Check sheet for the drawn part. Datum: minimum x, y, z corner. Units: mm. Coordinates: 2 decimals unless noted, no trailing zeros. Order: outer loops, then holes, each group sorted by start corner. A loop starts at its lowest first (then second) coordinate and runs counter-clockwise, first axis right, second up.
1. Gauge pin test, flat end, axial feed: pin 1 Ø2 at (x, y) = (8, 77) entering from -Z. Record the tip position at first contact, or that the pin passes through.
2. Cross-section at B-B (x = 24). Enter the section's corners in (y, z).
3. Cross-section at A-A (y = 27). Enter the section's corners in (x, z), then the cut area to 3 significant figures.
4. Thickness scan on line 1 (Y direction, x = 24, z = 2.7); line 2 (X direction, y = 27, z = 1.8); line 3 (Y direction, x = 20.5, z = 2.8). Record the ranges inside material, lowest first.
5. Cross-section at D-D (y = 86). Enter the section's corners in (x, z).
6. Cross-section at C-C (z = 0.8). Enter the section's corners in (x, y).
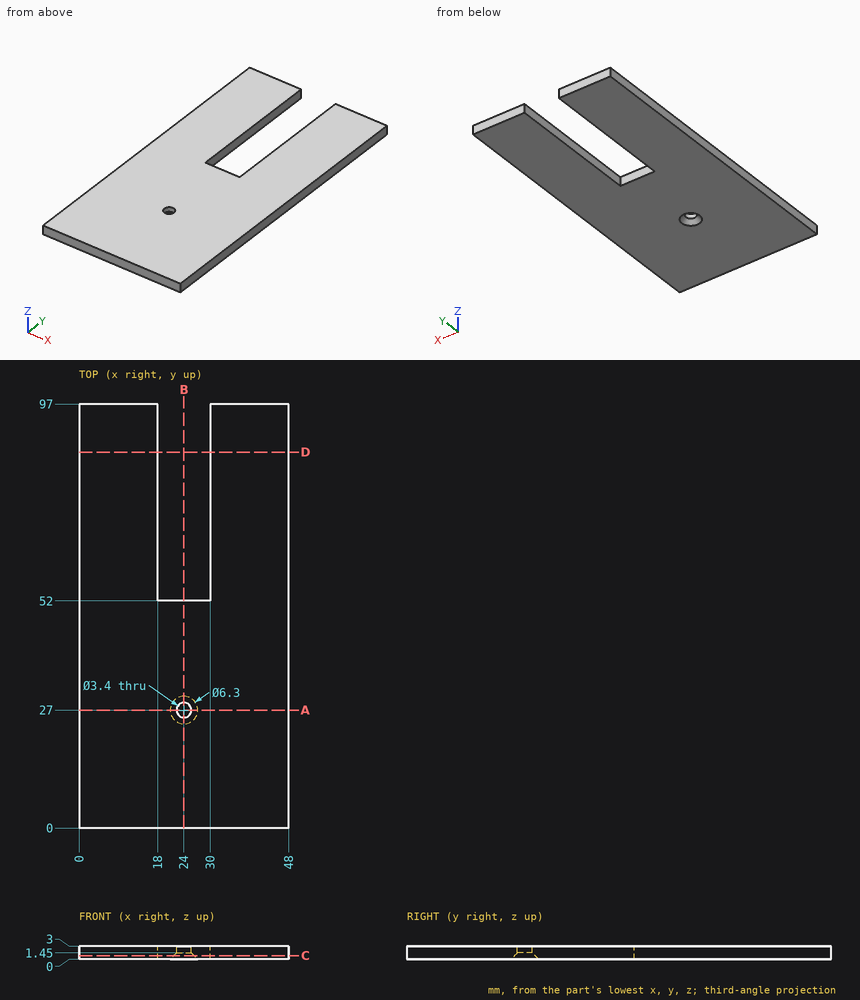
Data:
1. pin 1: stops at z = 0
2. outline: (0, 0) - (23.85, 0) - (25.3, 1.45) - (25.3, 3) - (0, 3) - close; (28.7, 1.45) - (30.15, 0) - (52, 0) - (52, 3) - (28.7, 3) - close
3. outline: (0, 0) - (20.85, 0) - (22.3, 1.45) - (22.3, 3) - (0, 3) - close; (25.7, 1.45) - (27.15, 0) - (48, 0) - (48, 3) - (25.7, 3) - close
3. area: 132 mm2
4. line 1: y = 0 to 25.3, 28.7 to 52
4. line 2: x = 0 to 22.3, 25.7 to 48
4. line 3: y = 0 to 52
5. outline: (0, 0) - (18, 0) - (18, 3) - (0, 3) - close; (30, 0) - (48, 0) - (48, 3) - (30, 3) - close
6. outline: (0, 0) - (48, 0) - (48, 97) - (30, 97) - (30, 52) - (18, 52) - (18, 97) - (0, 97) - close; hole circle Ø4.7 at (24, 27)
